from build123d import *

# Parameters (mm, degrees)
F0_W        = 76.2
F0_H        = 25.4
F1_DEPTH    = 11.43
F2_R        = 3.81
F3_DEPTH    = 6.35
F4_R        = 1.27
F5_W        = 25.4
F5_H        = 3.175
F6_DEPTH    = 9.525
F7_W        = 25.4
F7_H        = 3.175
F8_DEPTH    = 9.525
F9_T1_DEPTH = 52.1655609208
F10_R       = 1.27
F11_R       = 1.5875
F12_DEPTH   = 25.4
F13_R       = 1.5875
F14_DEPTH   = 25.4


# Not quite as in the source:
# - a fillet or chamfer that OpenCascade refuses, or shapes differently, is made with other operations: its cross-section is extruded or revolved along the edge and cut away or added


with BuildPart() as f1:
    # F0 (on Top) → F1 (new body)
    with BuildSketch(Plane.XY):
        with Locations((38.1, 12.7)):
            Rectangle(F0_W, F0_H)
    extrude(amount=F1_DEPTH)

    # F2 (on face) → F3 (cut)
    with BuildSketch(Plane.XY.offset(11.43)):
        with Locations((12.7, 12.7)):
            Circle(F2_R)
        with Locations((38.1, 12.7)):
            Circle(F2_R)
        with Locations((63.5, 12.7)):
            Circle(F2_R)
    extrude(amount=-F3_DEPTH, mode=Mode.SUBTRACT)

    # F4
    f4_edges = [f1.edges().sort_by_distance(p)[0] for p in [
        (38.1, 0, 11.43),
        (76.2, 12.7, 11.43),
        (38.1, 25.4, 11.43),
        (0, 12.7, 11.43),
    ]]
    fillet(f4_edges, radius=F4_R)

    # F5 (on face) → F6 (join)
    with BuildSketch(Plane.YZ.offset(76.2)):
        with Locations((12.7, 1.5875)):
            Rectangle(F5_W, F5_H)
    extrude(amount=F6_DEPTH)

    # F7 (on face) → F8 (join)
    with BuildSketch(Plane(origin=(0, 0, 0), x_dir=(0, -1, 0), z_dir=(-1, 0, 0))):
        with Locations((-12.7, 1.5875)):
            Rectangle(F7_W, F7_H)
    extrude(amount=F8_DEPTH)

    # F9: chamfer of 9.525 on 6 edges, made by hand

    # F9_s2 → F9_t1 (cut)
    with BuildSketch(Plane.XY.offset(-24.4952804604)):
        Polygon((0, 25.4), (-9.525, 15.875), (-9.525, 25.4), align=None)
        Polygon((76.2, 25.4), (85.725, 15.875), (85.725, 25.4), align=None)
        Polygon((85.725, 9.525), (76.2, 0), (85.725, 0), align=None)
        Polygon((-9.525, 9.525), (0, 0), (-9.525, 0), align=None)
    extrude(amount=F9_T1_DEPTH, mode=Mode.SUBTRACT)

    # F10
    f10_edges = [f1.edges().sort_by_distance(p)[0] for p in [
        (-4.7625, 4.7625, 3.175),
        (-9.525, 12.7, 3.175),
        (-4.7625, 20.6375, 3.175),
        (80.9625, 4.7625, 3.175),
        (85.725, 12.7, 3.175),
        (80.9625, 20.6375, 3.175),
    ]]
    fillet(f10_edges, radius=F10_R)

    # F11 (on face) → F12 (cut)
    with BuildSketch(Plane.XY.offset(3.175)):
        with Locations((-3.81, 12.7)):
            Circle(F11_R)
    extrude(amount=-F12_DEPTH, mode=Mode.SUBTRACT)

    # F13 (on face) → F14 (cut)
    with BuildSketch(Plane.XY.offset(3.175)):
        with Locations((80.01, 12.7)):
            Circle(F13_R)
    extrude(amount=-F14_DEPTH, mode=Mode.SUBTRACT)


solid = f1.part
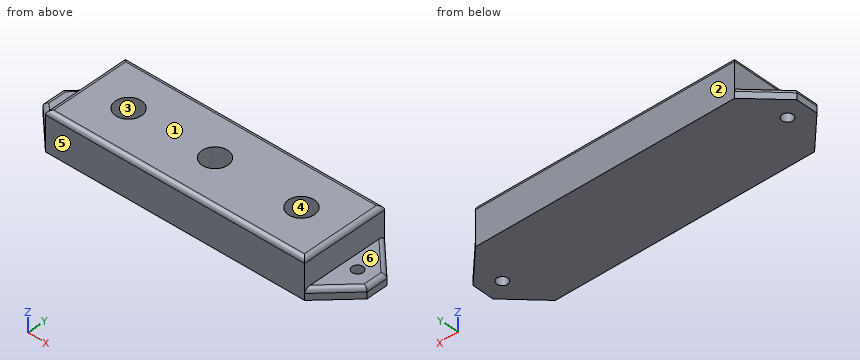
The listing builds one solid part. Answer for the finished solid, in the listing's coordinates (mm). Face numbers are marked on the shaded views. A direction names the side the tool comes from. Round coordinates to 2 decimals unless told otherwise and drop trailing zeros. Order: outer loops, then holes, each group sorted by start corner. A loop starts at its lowest first (then second) coordinate and runs counter-clockwise, first axis right, second up. Notation, with made-up numbers: M 47,3.5 L 82,3.5 A14 cw 82,30.5 Z; hole C 85,66.5 d11. An arc over 180 degrees is marked long. Answer in a Markdown table with one row per item. Add a question column.
1) The part is cut by section A-A on y = 12.7. Count the separate pieces of the cut face and the enclosed holes in it, plus the area to 3 significant figures.
2) The part is cut by section B-B on x = 12.7. Determine the outline of the cut face in (y, z).
3) Consider line 1 along Y through (x, z) = (12.7, 8.75); line 2 along Z through (x, y) = (36.5, 11); line 3 along X through (y, z) = (9.75, 6). Determine where each line is inside the solid, lowest interval first. Write a range as from..to.
4) Which of the six approach directions +Z, -Z, +X, -X, +Y, -Y give full straight-line access (tool end or side, diameter ignored) to the marked faces 4, 5 and 6?
5) The part is cut by section D-D on x = 40. Determine the outline of the cut face in (y, z).
6) Flat-ended cylindrical pins translate along their axes: pin 1 Ø1.9 at (x, y) = (80.01, 12.7) entering from -Z; pin 2 Ø4 at (x, y) = (80, 9) entering from +Z (3 decimals); pin 3 Ø6 at (x, y) = (12.7, 12.7) entering from +Z; pin 4 Ø8 at (x, y) = (61.5, 11) entering from -Z. Find the tip coordinate at first contact, or state that the pin passes through.
7) The part is cut by section C-C on z = 4. Determine the outline of the cut face in (x, y).
8) Determine the mould class of the marked faces 1, 2 and 3 for opening direction Y: pulls with the +Y half, pulls with the -Y half, needs draft (parallel to the pull), parting line crosses it, or undercut.
Findings below:
| question | item | result |
|---|---|---|
| 1 | separate pieces | 3 |
| 1 | enclosed holes | 0 |
| 1 | area | 765 mm² |
| 2 | outline | M 0,0 L 25.4,0 L 25.4,10.16 A1.27 ccw 24.13,11.43 L 16.51,11.43 L 16.51,5.08 L 8.89,5.08 L 8.89,11.43 L 1.27,11.43 A1.27 ccw 0,10.16 Z |
| 3 | line 1 | y = 0..8.89, 16.51..25.4 |
| 3 | line 2 | z = 0..5.08 |
| 3 | line 3 | x = 0..10.29, 15.11..35.69, 40.51..61.09, 65.91..76.2 |
| 4 | face 4 | +Z |
| 4 | face 5 | +Z, -Z, +X, -X, -Y |
| 4 | face 6 | +Z, +X, +Y, -Y |
| 5 | outline | M 0,0 L 25.4,0 L 25.4,10.16 A1.27 ccw 24.13,11.43 L 16,11.43 L 16,5.08 L 9.4,5.08 L 9.4,11.43 L 1.27,11.43 A1.27 ccw 0,10.16 Z |
| 6 | pin 1 | passes through |
| 6 | pin 2 | stops at z = 3.175 |
| 6 | pin 3 | stops at z = 5.08 |
| 6 | pin 4 | stops at z = 0 |
| 7 | outline | M 0,0 L 76.2,0 L 76.2,25.4 L 0,25.4 Z |
| 8 | face 1 | needs draft |
| 8 | face 2 | pulls with the +Y half |
| 8 | face 3 | undercut |
